CAD build for the part. Positions are in the model's coordinates, mm. Round coordinates to 2 decimals unless told otherwise and drop trailing zeros. Loops run counter-clockwise (first coordinate to the right, second up) from the corner with the lowest first, then second, coordinate; pieces in that order, holes last. Notation, with made-up numbers: M -11,31.25 L 14,31.25 A35 cw 14,66.25 Z; hole C 73,-1 d4. An arc over 180 degrees is marked long. Use one line per item in the form item = value.
from build123d import *

# Parameters (mm, degrees)
SKETCH_1_W          = 10
SKETCH_1_H          = 75
EXTRUDE_1_DEPTH     = 1.5
FILLET_1_R          = 2
SKETCH_3_R          = 1.5
CUT_EXTRUDE_1_DEPTH = 10


with BuildPart() as part:
    # 草图1 → 凸台-拉伸1 (new, symmetric)
    with BuildSketch(Plane.XY):
        Rectangle(SKETCH_1_W, SKETCH_1_H)
    extrude(amount=EXTRUDE_1_DEPTH, both=True)

    # 圆角1
    fillet_1_edges = [part.edges().sort_by_distance(p)[0] for p in [
        (0, -37.5, -1.5),
        (-5, 0, -1.5),
        (0, 37.5, -1.5),
        (5, 0, -1.5),
        (5, -37.5, 0),
        (-5, -37.5, 0),
        (-5, 37.5, 0),
        (5, 37.5, 0),
    ]]
    fillet(fillet_1_edges, radius=FILLET_1_R)

    # 草图3 → 切除-拉伸1 (cut)
    with BuildSketch(Plane.XY.offset(1.5)):
        with Locations((0, 31)):
            Circle(SKETCH_3_R)
        with Locations((0, -32.5)):
            Circle(SKETCH_3_R)
    extrude(amount=-CUT_EXTRUDE_1_DEPTH, mode=Mode.SUBTRACT)


solid = part.part
1. Probe line 1 along Y through (x, z) = (0, 0.8); line 2 along Y through (x, z) = (0, -0.8); line 3 along Z through (x, y) = (-3.25, 3.5). List the from-to ranges inside material, lowest first. Write a range as from..to.
Completed:
line_1 = -37.5..-34, -31..29.5, 32.5..37.5
line_2 = -37.02..-34, -31..29.5, 32.5..37.02
line_3 = -1.48..1.5
2. Cut at A-A on x = 0. Write the cut outline in (y, z), and give its area (3 significant figures).
Completed:
outline = M -37.5,0.5 A2 ccw -35.5,-1.5 L -34,-1.5 L -34,1.5 L -37.5,1.5 Z; M -31,-1.5 L 29.5,-1.5 L 29.5,1.5 L -31,1.5 Z; M 32.5,-1.5 L 35.5,-1.5 A2 ccw 37.5,0.5 L 37.5,1.5 L 32.5,1.5 Z
area = 205 mm2
3. Cut at B-B on y = -32.5. Write the cut outline in (x, z), and give its area (3 significant figures).
Completed:
outline = M -5,0.5 A2 ccw -3,-1.5 L -1.5,-1.5 L -1.5,1.5 L -5,1.5 Z; M 1.5,-1.5 L 3,-1.5 A2 ccw 5,0.5 L 5,1.5 L 1.5,1.5 Z
area = 19.3 mm2
4. Cut at C-C on y = -11.5. Write the cut outline in (x, z).
Completed:
outline = M -5,0.5 A2 ccw -3,-1.5 L 3,-1.5 A2 ccw 5,0.5 L 5,1.5 L -5,1.5 Z
5. Pull direction X, two halves, no side cores. Call faces 1 (the face through (-1.11, 32.01, 0.02)), 2 (the face through (4.43, -36.9, 1.01)), 3 (the face through (0, 0, -1.5)): +X half, -X half, draft (parallel to the pull), parting line (faces both ways), or undercut.
Completed:
face_1 = undercut
face_2 = +X half
face_3 = draft
6. Drop flat-ended pins along their axis: P1, Ø4, axis at x = 0, y = 31, coming from the +Z side; P2, Ø1, axis at y = -1.5, z = -1, coming from the +X side. Give the stop position or say it passes through.
Completed:
P1 = 1.5
P2 = 4.73
